from build123d import *

# Parameters (mm, degrees)
F0_R     = 0.191188
F1_DEPTH = 6.35
F2_SIZE  = 2.5146


with BuildPart() as f1:
    # F0 (on Top) → F1 (new body)
    with BuildSketch(Plane.XY):
        with BuildLine():
            Line((0.602884, -0.19939), (3.175, -0.19939))
            Line((3.175, -0.19939), (3.175, 0.19939))
            Line((3.175, 0.19939), (0.602884, 0.19939))
            ThreePointArc((0.602884, 0.19939), (0.44854, 0.449485), (0.19812, 0.603302))
            Line((0.19812, 0.603302), (0.19812, 3.175))
            Line((0.19812, 3.175), (-0.19812, 3.175))
            Line((-0.19812, 3.175), (-0.19812, 0.603302))
            ThreePointArc((-0.19812, 0.603302), (-0.44854, 0.449485), (-0.602884, 0.19939))
            Line((-0.602884, 0.19939), (-3.175, 0.19939))
            Line((-3.175, 0.19939), (-3.175, -0.19939))
            Line((-3.175, -0.19939), (-0.602884, -0.19939))
            ThreePointArc((-0.602884, -0.19939), (-0.44854, -0.449485), (-0.19812, -0.603302))
            Line((-0.19812, -0.603302), (-0.19812, -3.175))
            Line((-0.19812, -3.175), (0.19812, -3.175))
            Line((0.19812, -3.175), (0.19812, -0.603302))
            ThreePointArc((0.19812, -0.603302), (0.44854, -0.449485), (0.602884, -0.19939))
        make_face()
        Circle(F0_R, mode=Mode.SUBTRACT)
    extrude(amount=F1_DEPTH)

    # F2
    f2_edges = [f1.edges().sort_by_distance(p)[0] for p in [
        (0, -3.175, 6.35),
        (-3.175, 0, 6.35),
        (3.175, 0, 6.35),
        (0, 3.175, 6.35),
    ]]
    chamfer(f2_edges, length=F2_SIZE)


solid = f1.part
Work out the finished part from the listing and answer in its coordinate system (mm). A direction names the side the tool comes from. Give positions to 0.01 mm unless a question says otherwise; leave off trailing zeros. Write each loop counter-clockwise with the first axis right and the second up, starting at its lowest first coordinate (ties: lowest second). Pieces come first, ordered by that corner, then holes. Notation, with made-up numbers: M -40,-10 L 14,-10 A35 cw 14,23 Z; hole C 8.25,49.5 d10. An arc over 180 degrees is marked long. Answer as CSV lines item,"result".
Q1. A cutting plane is placed at C-C on z = 5.5. Write down the section's boundary in (x, y) (3 decimals).
A:
outline,"M -1.51,-0.199 L -0.603,-0.199 A0.635 ccw -0.198,-0.603 L -0.198,-1.51 L 0.198,-1.51 L 0.198,-0.603 A0.635 ccw 0.603,-0.199 L 1.51,-0.199 L 1.51,0.199 L 0.603,0.199 A0.635 ccw 0.198,0.603 L 0.198,1.51 L -0.198,1.51 L -0.198,0.603 A0.635 ccw -0.603,0.199 L -1.51,0.199 Z; hole C 0,0 d0.382"
Q2. A tool of negligible diameter and unlimited length cuts with its end or side. For faces 1 (the flat face through (0.198, -2, 2)), 2 (the flat face through (-2, 0.199, 2)), 3 (the flat face through (0.198, 2, 2)), 4 (the flat face through (-2, -0.199, 2)), from which of +Z, -Z, +X, -X, +Y, -Y can it reach the whole face along a straight path? Write none if from no direction.
A:
face 1,"+Z, -Z, +X, -Y"
face 2,"+Z, -Z, -X, +Y"
face 3,"+Z, -Z, +X, +Y"
face 4,"+Z, -Z, -X, -Y"
Q3. A cutting plane is placed at D-D on y = -1.5. Write down the section's boundary in (x, z), plus the area to 3 significant figures.
A:
outline,"M -0.2,0 L 0.2,0 L 0.2,5.51 L -0.2,5.51 Z"
area,"2.18 mm²"
Q4. Given P1, Ø1.5, axis at x = -2, z = 4.5, coming from the -Y side; P2, Ø0.8, axis at y = 2, z = 3, coming from the -X side; P3, Ø1.3, axis at y = -2.5, z = 4.5, coming from the +X side; P4, Ø2, axis at x = 1.5, y = 2, coming from the -Z side, each flat-ended and moving along its own axis, determine where each tip first touches the part or whether it passes through.
A:
P1,"stops at y = -0.2"
P2,"stops at x = -0.2"
P3,"stops at x = 0.2"
P4,"passes through"
Q5. Find the intervals of material crossed by probe 1 along Y at (x, z) = (0, 1.5) (3 decimals); probe 2 along Y at (x, z) = (1.25, 4.5); probe 3 along Y at (x, z) = (0, 4.75), in increasing order. Write a range as [from, to].
A:
probe 1,"y = [-3.175, -0.191], [0.191, 3.175]"
probe 2,"y = [-0.2, 0.2]"
probe 3,"y = [-2.26, -0.19], [0.19, 2.26]"
Q6. A cutting plane is placed at A-A on y = 0. Write down the section's boundary in (x, z) (3 decimals), plus the area to 3 significant figures.
A:
outline,"M -3.175,0 L -0.191,0 L -0.191,6.35 L -0.66,6.35 L -3.175,3.835 Z; M 0.191,0 L 3.175,0 L 3.175,3.835 L 0.66,6.35 L 0.191,6.35 Z"
area,"31.6 mm²"
